from build123d import *

# Parameters (mm, degrees)
EXTRUDE_1_DEPTH     = 1.5
FILLET_1_R          = 1
SKETCH_3_R          = 0.75
CUT_EXTRUDE_1_DEPTH = 4
SKETCH_4_R          = 0.75
CUT_EXTRUDE_2_DEPTH = 4
SKETCH_5_R          = 0.75
CUT_EXTRUDE_3_DEPTH = 4
CUT_EXTRUDE_6_DEPTH = 4


with BuildPart() as part:
    # 草图1 → 凸台-拉伸1 (new body, symmetric)
    with BuildSketch(Plane.XY):
        Polygon((0, 10), (10.6, 10), (10.6, 12.5), (30.6, 12.5), (30.6, 10), (36.6, 10), (36.6, 7.55), (30.6, 7.55), (30.6, 5), (34.6, 5), (34.6, -5), (30.6, -5), (30.6, -7.55), (36.6, -7.55), (36.6, -10), (30.6, -10), (30.6, -12.5), (10.6, -12.5), (10.6, -10), (0, -10), align=None)
        Polygon((6.6, 5), (10.6, 5), (10.6, 7.55), (2.5, 7.55), (2.5, -7.55), (10.6, -7.55), (10.6, -5), (6.6, -5), align=None, mode=Mode.SUBTRACT)
    extrude(amount=EXTRUDE_1_DEPTH, both=True)

    # 圆角1
    fillet_1_edges = [part.edges().sort_by_distance(p)[0] for p in [
        (0, 10, 0),
        (36.6, 10, 0),
        (34.6, 5, 0),
        (34.6, -5, 0),
        (36.6, -10, 0),
        (0, -10, 0),
        (6.6, -5, 0),
        (6.6, 5, 0),
    ]]
    fillet(fillet_1_edges, radius=FILLET_1_R)

    # 草图3 → 切除-拉伸1 (cut, through all)
    with BuildSketch(Plane.XY.offset(1.5)):
        with Locations((9.85, 7.55)):
            Circle(SKETCH_3_R)
        with Locations((9.85, -7.55)):
            Circle(SKETCH_3_R)
        with Locations((31.35, 7.55)):
            Circle(SKETCH_3_R)
        with Locations((30.6, 5.75)):
            Circle(SKETCH_3_R)
        with Locations((30.6, -5.75)):
            Circle(SKETCH_3_R)
        with Locations((31.35, -7.55)):
            Circle(SKETCH_3_R)
        with Locations((10.6, 5.75)):
            Circle(SKETCH_3_R)
        with Locations((10.6, -5.75)):
            Circle(SKETCH_3_R)
    extrude(amount=-CUT_EXTRUDE_1_DEPTH, mode=Mode.SUBTRACT)

    # 草图4 → 切除-拉伸2 (cut, through all)
    with BuildSketch(Plane.XY.offset(1.5)):
        with Locations((10.6, 10.75)):
            Circle(SKETCH_4_R)
        with Locations((30.6, 10.75)):
            Circle(SKETCH_4_R)
        with Locations((10.6, -10.75)):
            Circle(SKETCH_4_R)
        with Locations((30.6, -10.75)):
            Circle(SKETCH_4_R)
    extrude(amount=-CUT_EXTRUDE_2_DEPTH, mode=Mode.SUBTRACT)

    # 草图5 → 切除-拉伸3 (cut, through all)
    with BuildSketch(Plane.XY.offset(1.5)):
        with Locations((2.5, 6.8)):
            Circle(SKETCH_5_R)
        with Locations((2.5, -6.8)):
            Circle(SKETCH_5_R)
    extrude(amount=-CUT_EXTRUDE_3_DEPTH, mode=Mode.SUBTRACT)

    # 草图8 → 切除-拉伸6 (cut, through all)
    with BuildSketch(Plane.XY.offset(1.5)):
        Polygon((13.6, -12.5), (14.300207538, -11.5), (26.899792462, -11.5), (27.6, -12.5), align=None)
    cut_extrude_6 = extrude(amount=-CUT_EXTRUDE_6_DEPTH, mode=Mode.SUBTRACT)

    # 镜向2: 切除-拉伸6 across plane
    add(cut_extrude_6.mirror(Plane.ZX), mode=Mode.SUBTRACT)


solid = part.part
Model file for the job. Use its own axes, mm. A direction names the side the tool comes from. Round coordinates to 2 decimals unless told otherwise and drop trailing zeros. Order: outer loops, then holes, each group sorted by start corner. A loop starts at its lowest first (then second) coordinate and runs counter-clockwise, first axis right, second up.
(1) 3-axis set-ups, long thin cutter, end or side, ignore diameter. For faces 1 (the face through (34, 7.55, 0)), 2 (the face through (9, -5, 0)), 3 (the face through (13.945, 12.007, 0.021)), 4 (the face through (30.6, 12, 0)), 5 (the face through (27.245, -11.993, 0.021)): which of +Z, -Z, +X, -X, +Y, -Y reach the whole face in a straight line?
(2) Pull direction Y, two halves, no side cores. Call faces 6 (the face through (36.315, -9.699, 0.021)), 7 (the face through (12, 12.5, 0)), 8 (the face through (34.315, 4.699, -0.021)): released by +Y, released by -Y, zero draft, split by the parting line, or undercut.
(3) Band-saw the part on C-C (x = 5.5). List the corners of the cut face in (y, z), then the cut area to 3 significant figures.
(4) Band-saw the part on A-A (x = 31.35). List the corners of the cut face in (y, z), then the cut area to 3 significant figures.
(5) Drill centre lines: line 1 (X direction, y = 1.5, z = -0.05); line 2 (Y direction, x = 5.5, z = 0.4); line 3 (Y direction, x = 9, z = 1.15). Where is each one in solid material? Low to high.
(6) Band-saw the part on B-B (y = 1). List the corners of the cut face in (x, z).
(7) Band-saw the part on D-D (x = 19). List the corners of the cut face in (y, z).
(8) Pin check, flat tips, straight feed: pin 1 (1.1 mm diameter, centred on y = -12, z = -0.5, fed in from -X); pin 2 (0.9 mm diameter, centred on x = 4, z = 0.5, fed in from -Y); pin 3 (0.8 mm diameter, centred on y = 12, z = -0.5, fed in from +X). Stop position of each tip, or through.
Verdict:
1. face 1: +Z, -Z, +X
1. face 2: +Z, -Z
1. face 3: +Z, -Z, +Y
1. face 4: +Z, -Z, +X, +Y
1. face 5: +Z, -Z, -Y
2. face 6: released by -Y
2. face 7: released by +Y
2. face 8: undercut
3. outline: (-10, -1.5) - (-7.55, -1.5) - (-7.55, 1.5) - (-10, 1.5) - close; (7.55, -1.5) - (10, -1.5) - (10, 1.5) - (7.55, 1.5) - close
3. area: 14.7 mm2
4. outline: (-10, -1.5) - (-8.3, -1.5) - (-8.3, 1.5) - (-10, 1.5) - close; (-5, -1.5) - (5, -1.5) - (5, 1.5) - (-5, 1.5) - close; (8.3, -1.5) - (10, -1.5) - (10, 1.5) - (8.3, 1.5) - close
4. area: 40.2 mm2
5. line 1: x = 0 to 2.5, 6.6 to 34.6
5. line 2: y = -10 to -7.55, 7.55 to 10
5. line 3: y = -10 to -7.55, -5 to 5, 7.55 to 10
6. outline: (0, -1.5) - (2.5, -1.5) - (2.5, 1.5) - (0, 1.5) - close; (6.6, -1.5) - (34.6, -1.5) - (34.6, 1.5) - (6.6, 1.5) - close
7. outline: (-11.5, -1.5) - (11.5, -1.5) - (11.5, 1.5) - (-11.5, 1.5) - close
8. pin 1: stops at x = 10.6
8. pin 2: stops at y = -10
8. pin 3: stops at x = 30.6
